```python
from build123d import *

# Parameters (mm, degrees)
ESTRUSIONE_ESTRUSIONE1_DEPTH  = 14.6
SCHIZZO2_W                    = 64
SCHIZZO2_H                    = 3
ESTRUSIONE_ESTRUSIONE2_DEPTH  = 14.7
ESTRUSIONE_ESTRUSIONE3_DEPTH  = 11.3
ESTRUSIONE_ESTRUSIONE4_DEPTH  = 14.9
SCHIZZO6_W                    = 64
SCHIZZO6_H                    = 3.1
ESTRUSIONE_ESTRUSIONE5_DEPTH  = 13
ESTRUSIONE_ESTRUSIONE8_START  = -64
ESTRUSIONE_ESTRUSIONE8_DEPTH  = 64
ESTRUSIONE_ESTRUSIONE9_DEPTH  = 14.6
ESTRUSIONE_ESTRUSIONE13_DEPTH = 14.7
ESTRUSIONE_ESTRUSIONE14_START = -3.1
ESTRUSIONE_ESTRUSIONE14_DEPTH = 3.1
TAGLIO_ESTRUSIONE3_DEPTH      = 15
TAGLIO_ESTRUSIONE4_REACH      = 94.756
ESTRUSIONE_ESTRUSIONE15_DEPTH = 2


with BuildPart() as part:
    # Schizzo1 → Estrusione-Estrusione1 (new body)
    with BuildSketch(Plane.XY):
        with BuildLine():
            Line((0, 30), (0, 0))
            Line((0, 0), (1.1, 0))
            Line((1.1, 0), (1.1, -6))
            Line((1.1, -6), (83.6, -6))
            Line((83.6, -6), (83.6, 0))
            ThreePointArc((83.6, 0), (77.157447993, 15.380640119), (66.7, 28.36957188))
            Line((66.7, 28.36957188), (62.855201518, 23.378827984))
            ThreePointArc((62.855201518, 23.378827984), (54.861139367, 22.342020228), (53.824331611, 30.336082379))
            Line((53.824331611, 30.336082379), (57.669130093, 35.326826275))
            ThreePointArc((57.669130093, 35.326826275), (43.389650216, 41.844502061), (27.902688632, 44.401387681))
            Line((27.902688632, 44.401387681), (0, 30))
        make_face()
    extrude(amount=ESTRUSIONE_ESTRUSIONE1_DEPTH)

    # Schizzo2 → Estrusione-Estrusione2 (add)
    with BuildSketch(Plane(origin=(0, 0, 0), x_dir=(-1, 0, 0), z_dir=(0, 0, -1))):
        with Locations((-33.1, -4.5)):
            Rectangle(SCHIZZO2_W, SCHIZZO2_H)
    extrude(amount=ESTRUSIONE_ESTRUSIONE2_DEPTH)

    # Schizzo4 → Estrusione-Estrusione3 (add)
    with BuildSketch(Plane.XY.offset(14.6)):
        Polygon((1.1, -6), (12.4, -6), (1.1, -11), align=None)
    extrude(amount=-ESTRUSIONE_ESTRUSIONE3_DEPTH)

    # Schizzo5 → Estrusione-Estrusione4 (add)
    with BuildSketch(Plane(origin=(0, 0, 3.3), x_dir=(-1, 0, 0), z_dir=(0, 0, -1))):
        Polygon((-1.1, -6), (-33.8, -6), (-1.1, -19), align=None)
    extrude(amount=ESTRUSIONE_ESTRUSIONE4_DEPTH)

    # Schizzo6 → Estrusione-Estrusione5 (add)
    with BuildSketch(Plane.XZ.offset(6)):
        with Locations((33.1, -13.15)):
            Rectangle(SCHIZZO6_W, SCHIZZO6_H)
    extrude(amount=ESTRUSIONE_ESTRUSIONE5_DEPTH)

    # Schizzo7 → Estrusione-Estrusione8 (add)
    with BuildSketch(Plane(origin=(65.1, 0, 0), x_dir=(0, 0, -1), z_dir=(1, 0, 0)).offset(ESTRUSIONE_ESTRUSIONE8_START)):
        Polygon((14.7, -19), (14.7, -22.05), (11.6, -19), align=None)
    extrude(amount=ESTRUSIONE_ESTRUSIONE8_DEPTH)

    # Schizzo9 → Estrusione-Estrusione9 (add)
    with BuildSketch(Plane.XY):
        Polygon((83.6, -6), (65.1, -6), (83.6, -22), align=None)
    extrude(amount=ESTRUSIONE_ESTRUSIONE9_DEPTH)

    # Schizzo16 → Estrusione-Estrusione13 (add)
    with BuildSketch(Plane(origin=(0, 0, 0), x_dir=(-1, 0, 0), z_dir=(0, 0, -1))):
        Polygon((-65.1, -3), (-83.6, -19), (-83.6, -22), (-65.1, -6), align=None)
    extrude(amount=ESTRUSIONE_ESTRUSIONE13_DEPTH)

    # Schizzo17 → Estrusione-Estrusione14 (add)
    with BuildSketch(Plane(origin=(0, 0, -14.7), x_dir=(-1, 0, 0), z_dir=(0, 0, -1)).offset(ESTRUSIONE_ESTRUSIONE14_START)):
        Polygon((-65.1, -6), (-65.1, -22.05), (-83.6, -22), align=None)
    extrude(amount=ESTRUSIONE_ESTRUSIONE14_DEPTH)

    # Schizzo18 → Taglio-Estrusione3 (cut)
    with BuildSketch(Plane.ZY.offset(-65.1)):
        Polygon((-11.6, -22.05), (-11.6, -19), (-14.7, -22.05), align=None)
    extrude(amount=-TAGLIO_ESTRUSIONE3_DEPTH, mode=Mode.SUBTRACT)

    # Taglio-Estrusione4: up to this face of the body (flat: up to its plane)
    taglio_estrusione4_end = Plane(part.part.faces().sort_by_distance((74.35, -14, 1.5))[0])
    # Schizzo20 → Taglio-Estrusione4 (cut, up to the picked face)
    with BuildSketch(Plane.ZY.offset(-80.1), mode=Mode.PRIVATE) as taglio_estrusione4_sk1:
        Polygon((-11.6, -22.009459459), (-11.6, -19), (-14.65879486, -22.009459459), align=None)
    taglio_estrusione4_tool1 = split(extrude(taglio_estrusione4_sk1.sketch, amount=-TAGLIO_ESTRUSIONE4_REACH, mode=Mode.PRIVATE), bisect_by=taglio_estrusione4_end, keep=Keep.BOTH, mode=Mode.PRIVATE)
    add(taglio_estrusione4_tool1.solids().sort_by(Axis((80.1, -21.006306, -12.619598), (1, 0, 0)))[0], mode=Mode.SUBTRACT)

    # Schizzo22 → Loft3 section 0
    with BuildSketch(Plane(origin=(0, 0, -14.7), x_dir=(-1, 0, 0), z_dir=(0, 0, -1))):
        with BuildLine():
            Line((-65.1, -6), (-62.68232007, -6))
            Line((-62.68232007, -6), (-83.6, -22))
            Line((-83.6, -22), (-65.1, -6))
        make_face()
    # Schizzo23 → Loft3 section 1
    with BuildSketch(Plane.XY.offset(14.6)):
        with BuildLine():
            Line((65.1, -6), (83.6, -22))
            Line((83.6, -22), (63.891160035, -6))
            Line((63.891160035, -6), (65.1, -6))
        make_face()
    loft()

    # Schizzo19 → Estrusione-Estrusione15 (add)
    with BuildSketch(Plane.XY.offset(14.6)):
        with BuildLine():
            Line((0, 30), (10.3, 35.316129032))
            Line((10.3, 35.316129032), (18.7, 9.316129032))
            Line((18.7, 9.316129032), (31.7, 0))
            ThreePointArc((31.7, 0), (33.987904201, -2.59259381), (33.4, -6))
            Line((33.4, -6), (12.4, -6))
            Line((12.4, -6), (1.1, -11))
            Line((1.1, -11), (1.1, 0))
            Line((1.1, 0), (0, 0))
            Line((0, 0), (0, 30))
        make_face()
    extrude(amount=ESTRUSIONE_ESTRUSIONE15_DEPTH)


solid = part.part
```
Work out the finished part from the listing and answer in its coordinate system (mm). A direction names the side the tool comes from. Give positions to 0.01 mm unless a question says otherwise; leave off trailing zeros. Loops run counter-clockwise (first coordinate to the right, second up) from the corner with the lowest first, then second, coordinate; pieces in that order, holes last. Notation, with made-up numbers: (34.25, -7.75) - (50.25, -7.75) arc R30 cw to (50.25, 20.25) - close; hole circle Ø2 at (52, 83). An arc over 180 degrees is marked (long way). Use CSV: the item, a comma, the result in double quotes. Start each with the question number.
(1) Find section B-B, the plane x = 16. Determine the outline of the cut face in (y, z).
(2) Find section C-C, the plane y = 1. Determine the outline of the cut face in (x, z), plus the area to 3 significant figures.
(3) Find section D-D, the plane x = 7. Determine the outline of the cut face in (y, z).
(4) A tool of negligible diameter and unlimited length cuts with its end or side. For faces 1 (the face through (34, -3, -7)), 2 (the face through (1.1, -9, -3)), 3 (the face through (64.8, 25.9, 7.2)), 4 (the face through (14, -11, 3.3)), from which of +Z, -Z, +X, -X, +Y, -Y can it reach the whole face along a straight path? Write none if from no direction.
(5) Determine the mould class of faces 5 (the face through (55.72, 32.8, 7.2)), 6 (the face through (74.22, -10.89, -7.25)), 7 (the face through (33.974, -2.545, 15.586)) for opening direction Y: released by +Y, released by -Y, zero draft, split by the parting line, or undercut.
(6) Each of these flat-tipped pins is pushed along its axis until it touches: pin 1 (4 mm diameter, centred on x = 31.5, y = -15.5, fed in from +Z); pin 2 (7.5 mm diameter, centred on x = 19, z = -3.5, fed in from +Y); pin 3 (5 mm diameter, centred on x = 72.5, y = -5.5, fed in from +Z). Where does it stop, or does it pass through?
(7) Find section A-A, the plane y = 25. Determine the outline of the cut face in (x, z).
(8) Find the intervals of material crossed by L1, parallel to Y at x = 48, z = -8.5; L2, parallel to Z at x = 70, y = 24; L3, parallel to Z at x = 26, y = -13.5, in increasing order.
Results found:
1,outline,"(-22.05, -14.7) - (-3, -14.7) - (-3, 0) - (38.26, 0) - (38.26, 14.6) - (17.67, 14.6) - (17.67, 16.6) - (-6, 16.6) - (-6, 3.3) - (-13.08, 3.3) - (-13.08, -11.6) - (-19, -11.6) - close"
2,outline,"(0, 0) - (83.33, 0) - (83.33, 14.6) - (30.3, 14.6) - (30.3, 16.6) - (0, 16.6) - close"
2,area,"1,280 mm^2"
3,outline,"(-22.05, -14.7) - (-3, -14.7) - (-3, 0) - (33.61, 0) - (33.61, 16.6) - (-8.39, 16.6) - (-8.39, 3.3) - (-16.65, 3.3) - (-16.65, -11.6) - (-19, -11.6) - close"
4,face 1,"-Z, +X, -X, +Y"
4,face 2,"+Z, -Z, -X, -Y"
4,face 3,"+Z, -Z, +Y"
4,face 4,"+Z, -Y"
5,face 5,"undercut"
5,face 6,"released by +Y"
5,face 7,"split by the parting line"
6,pin 1,"z = -11.6"
6,pin 2,"y = 40.5"
6,pin 3,"z = 14.6"
7,outline,"(0, 0) - (52.95, 0) - (52.95, 14.6) - (13.63, 14.6) - (13.63, 16.6) - (0, 16.6) - close; (64.1, 0) - (70.02, 0) - (70.02, 14.6) - (64.1, 14.6) - close"
8,L1,"-6 to -3"
8,L2,"0 to 14.6"
8,L3,"-14.7 to -11.6"
